Read the model definition and answer for the solid it produces. Units are mm, in the model's axes. Face numbers are marked on the shaded views. A direction names the side the tool comes from. Coordinates: 2 decimals unless noted, no trailing zeros. Loops run counter-clockwise (first coordinate to the right, second up) from the corner with the lowest first, then second, coordinate; pieces in that order, holes last.
Autodesk Fusion 360 part; units mm, degrees
sketch "草图1" plane through (0, 0, 0) normal (0, 0, 1) x (1, 0, 0)
  line L0 (-83.7376, 48.3346) -> (-83.7376, -57.8018)
  line L1 (100, -57.8018) -> (-83.7376, -57.8018)
  line L2 (99.9425, 14.822) -> (-83.7376, 48.3346)
  line L3 (99.9425, 14.822) -> (99.9425, -57.8018)
  line L4 (-75.3044, 2.9706) -> (90.6956, 2.9706)
  line L5 (90.6956, 2.9706) -> (90.6956, -51.4889)
  line L6 (90.6956, -51.4889) -> (-75.3044, -51.4889)
  line L7 (-75.3044, -51.4889) -> (-75.3044, 2.9706)
  dimension "d1" = 166
extrude "拉伸1" add sketch "草图1" along normal blind 20 contours L0 L1 L2 L3 | L4 L5 L6 L7
sketch "草图2" plane through (0, 0, 20) normal (0, 0, 1) x (-1, 0, 0)
  line L0 (83.7376, -48.3346) -> (83.7376, 57.8018)
  line L1 (83.7376, 57.8018) -> (-99.9425, 57.8018)
  line L2 (-99.9425, 57.8018) -> (-99.9425, -14.822)
  line L3 (-99.9425, -14.822) -> (83.7376, -48.3346)
  line L4 (75, -5) -> (-90, -5)
  line L5 (-90, -5) -> (-90, 50)
  line L6 (-90, 50) -> (75, 50)
  line L7 (75, 50) -> (75, -5)
extrude "拉伸2" cut sketch "草图2" against normal blind 15 contours L4 L5 L6 L7
sketch "草图3" plane through (0, 0, 20) normal (0, 0, 1) x (-1, 0, 0)
  line L0 (-90, -5) -> (-90, 50)
  line L1 (-90, 50) -> (75, 50)
  line L2 (75, 50) -> (75, -5)
  line L3 (75, -5) -> (-90, -5)
  line L4 (83.7376, -48.3346) -> (83.7376, 57.8018)
  line L5 (83.7376, 57.8018) -> (-99.9425, 57.8018)
  line L6 (-99.9425, 57.8018) -> (-99.9425, -14.822)
  line L7 (-99.9425, -14.822) -> (83.7376, -48.3346)
  line L8 (67.985, -5) -> (60.985, -5)
  line L9 (60.985, -5) -> (60.985, 26)
  line L10 (60.985, 26) -> (67.985, 26)
  line L11 (67.985, 26) -> (67.985, -5)
  line L12 (67.985, -5) -> (60.985, -5)
  line L13 (67.985, 26) -> (67.985, -5)
  line L14 (60.985, 26) -> (67.985, 26)
  line L15 (60.985, -5) -> (60.985, 26)
  line L16 (55.5549, 26) -> (55.5549, -5)
  line L17 (55.5549, -5) -> (48.5549, -5)
  line L18 (48.5549, -5) -> (48.5549, 26)
  line L19 (48.5549, 26) -> (55.5549, 26)
  line L20 (55.5549, 26) -> (55.5549, -5)
  line L21 (48.5549, 26) -> (55.5549, 26)
  line L22 (48.5549, -5) -> (48.5549, 26)
  line L23 (55.5549, -5) -> (48.5549, -5)
  line L24 (36.7829, -5) -> (29.7829, -5)
  line L25 (36.7829, 26) -> (36.7829, -5)
  line L26 (29.7829, 26) -> (36.7829, 26)
  line L27 (29.7829, -5) -> (29.7829, 26)
  line L28 (24.3528, 26) -> (24.3528, -5)
  line L29 (17.3528, 26) -> (24.3528, 26)
  line L30 (17.3528, -5) -> (17.3528, 26)
  line L31 (24.3528, -5) -> (17.3528, -5)
  line L32 (11.4154, 26) -> (11.4154, -5)
  line L33 (4.4154, -5) -> (4.4154, 26)
  line L34 (11.4154, -5) -> (4.4154, -5)
  line L35 (4.4154, 26) -> (11.4154, 26)
  line L36 (-52.6472, -5) -> (-59.6472, -5)
  line L37 (-21.4451, 26) -> (-21.4451, -5)
  line L38 (-9.015, -5) -> (-16.015, -5)
  line L39 (-28.4451, 26) -> (-21.4451, 26)
  line L40 (-28.4451, 26) -> (-21.4451, 26)
  line L41 (-40.2171, 26) -> (-40.2171, -5)
  line L42 (-40.2171, -5) -> (-47.2171, -5)
  line L43 (-72.5846, -5) -> (-72.5846, 26)
  line L44 (-47.2171, 26) -> (-40.2171, 26)
  line L45 (-47.2171, -5) -> (-47.2171, 26)
  line L46 (-52.6472, 26) -> (-52.6472, -5)
  line L47 (-65.5846, 26) -> (-65.5846, -5)
  line L48 (-9.015, 26) -> (-9.015, -5)
  line L49 (-16.015, 26) -> (-9.015, 26)
  line L50 (-21.4451, -5) -> (-28.4451, -5)
  line L51 (-28.4451, -5) -> (-28.4451, 26)
  line L52 (-16.015, -5) -> (-16.015, 26)
  line L53 (-28.4451, -5) -> (-28.4451, 26)
  line L54 (-9.015, -5) -> (-16.015, -5)
  line L55 (-16.015, 26) -> (-9.015, 26)
  line L56 (-72.5846, 26) -> (-65.5846, 26)
  line L57 (-65.5846, -5) -> (-72.5846, -5)
  line L58 (-21.4451, 26) -> (-21.4451, -5)
  line L59 (-9.015, 26) -> (-9.015, -5)
  line L60 (-21.4451, -5) -> (-28.4451, -5)
  line L61 (-59.6472, 26) -> (-52.6472, 26)
  line L62 (-59.6472, -5) -> (-59.6472, 26)
  line L63 (-16.015, -5) -> (-16.015, 26)
  line L64 (-82.7432, 26.3749) -> (-82.7432, -4.6251)
  line L65 (-89.7432, 26.3749) -> (-82.7432, 26.3749)
  line L66 (-89.7432, -4.6251) -> (-89.7432, 26.3749)
  line L67 (-82.9307, -4.8125) -> (-89.9307, -4.8125)
  point P0 (-77, 0)
  dimension "d6" = 7
  dimension "d7" = 31
  dimension "d8" = 7
  dimension "d9" = 31
  dimension "d10" = 7
  dimension "d11" = 31
  dimension "d12" = 7
  dimension "d13" = 31
  dimension "d14" = 7
  dimension "d15" = 31
  dimension "d16" = 31
  dimension "d17" = 7
  dimension "d18" = 31
  dimension "d19" = 7
  dimension "d22" = -77
  dimension "d23" = 0
  dimension "d24" = 7
  dimension "d25" = 31
  dimension "d26" = 7
extrude "拉伸3" add sketch "草图3" against normal blind 15 contours L3 L43 L47 L56 L57 | L3 L36 L46 L61 L62 | L3 L8 L9 L10 L11 L12 L13 L14 L15 | L3 L41 L42 L44 L45 | L3 L16 L17 L18 L19 L20 L21 L22 L23 | L3 L37 L39 L40 L50 L51 L53 L58 L60 | L3 L24 L25 L26 L27 | L3 L38 L48 L49 L52 L54 L55 L59 L63 | L3 L28 L29 L30 L31 | L3 L32 L33 L34 L35
sketch "草图4" plane through (0, 0, 20) normal (0, 0, 1) x (-1, 0, 0)
  line L0 (-90, -5) -> (-90, 50)
  line L1 (-90, 50) -> (75, 50)
  line L2 (75, 50) -> (75, -5)
  line L3 (75, -5) -> (67.985, -5)
  line L4 (67.985, -5) -> (67.985, 26)
  line L5 (67.985, 26) -> (60.985, 26)
  line L6 (60.985, 26) -> (60.985, -5)
  line L7 (60.985, -5) -> (55.5549, -5)
  line L8 (55.5549, -5) -> (55.5549, 26)
  line L9 (55.5549, 26) -> (48.5549, 26)
  line L10 (48.5549, 26) -> (48.5549, -5)
  line L11 (48.5549, -5) -> (36.7829, -5)
  line L12 (36.7829, -5) -> (36.7829, 26)
  line L13 (36.7829, 26) -> (29.7829, 26)
  line L14 (29.7829, 26) -> (29.7829, -5)
  line L15 (29.7829, -5) -> (24.3528, -5)
  line L16 (24.3528, -5) -> (24.3528, 26)
  line L17 (24.3528, 26) -> (17.3528, 26)
  line L18 (17.3528, 26) -> (17.3528, -5)
  line L19 (17.3528, -5) -> (11.4154, -5)
  line L20 (11.4154, -5) -> (11.4154, 26)
  line L21 (11.4154, 26) -> (4.4154, 26)
  line L22 (4.4154, 26) -> (4.4154, -5)
  line L23 (4.4154, -5) -> (-9.015, -5)
  line L24 (-9.015, -5) -> (-9.015, 26)
  line L25 (-9.015, 26) -> (-16.015, 26)
  line L26 (-16.015, 26) -> (-16.015, -5)
  line L27 (-16.015, -5) -> (-21.4451, -5)
  line L28 (-21.4451, -5) -> (-21.4451, 26)
  line L29 (-21.4451, 26) -> (-28.4451, 26)
  line L30 (-28.4451, 26) -> (-28.4451, -5)
  line L31 (-28.4451, -5) -> (-40.2171, -5)
  line L32 (-40.2171, -5) -> (-40.2171, 26)
  line L33 (-40.2171, 26) -> (-47.2171, 26)
  line L34 (-47.2171, 26) -> (-47.2171, -5)
  line L35 (-47.2171, -5) -> (-52.6472, -5)
  line L36 (-52.6472, -5) -> (-52.6472, 26)
  line L37 (-52.6472, 26) -> (-59.6472, 26)
  line L38 (-59.6472, 26) -> (-59.6472, -5)
  line L39 (-59.6472, -5) -> (-65.5846, -5)
  line L40 (-65.5846, -5) -> (-65.5846, 26)
  line L41 (-65.5846, 26) -> (-72.5846, 26)
  line L42 (-72.5846, 26) -> (-72.5846, -5)
  line L43 (-72.5846, -5) -> (-90, -5)
  line L44 (83.7376, -48.3346) -> (83.7376, 57.8018)
  line L45 (83.7376, 57.8018) -> (-99.9425, 57.8018)
  line L46 (-99.9425, 57.8018) -> (-99.9425, -14.822)
  line L47 (-99.9425, -14.822) -> (83.7376, -48.3346)
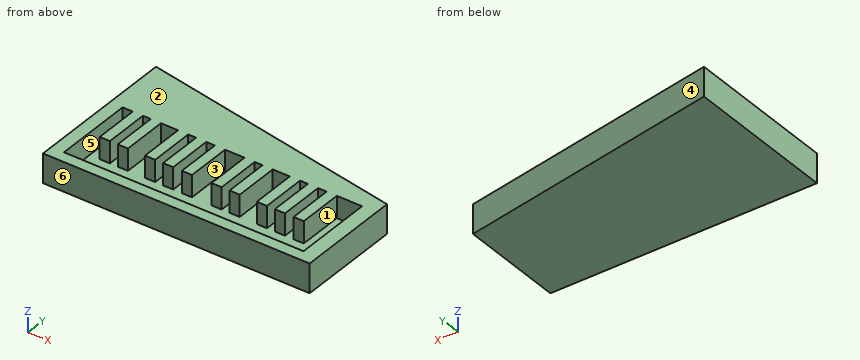
Q1. A cutting plane is placed at C-C (y = 25). Give the vertices of the cut face in (x, z), then the cut area to 3 significant figures.
Findings below:
outline: (-83.74, 0) - (44.16, 0) - (44.16, 20) - (-83.74, 20) - close
area: 2,560 mm2
Q2. A flat-ended cylindrical pin translates along its axis: pin 1 Ø1.5 at (x, z) = (-27.5, 5) entering from +Y. Find the tip coordinate at first contact, or state that the pin passes through.
Findings below:
pin 1: stops at y = 38.21
Q3. Which of the six approach directions +Z, -Z, +X, -X, +Y, -Y give full straight-line access (tool end or side, diameter ignored) to the marked faces 1 and 2?
Findings below:
face 1: +Z
face 2: +Z, +X, -X, +Y, -Y
Q4. Straight lines are drawn through the part: probe 1 along X at (y, z) = (-48, 5.25); probe 2 along Z at (x, y) = (38, 2.5); probe 3 along Y at (x, z) = (65.5, 18.75). For each, find the intervals that lie inside material, in ascending order.
Findings below:
probe 1: x = -83.74 to -75, 90 to 99.94
probe 2: z = 0 to 5
probe 3: y = -57.8 to -50, 5 to 21.11
Q5. A cutting plane is placed at B-B (x = -32). Give the vertices of the cut face in (y, z).
Findings below:
outline: (-57.8, 0) - (38.9, 0) - (38.9, 20) - (-26, 20) - (-26, 5) - (-50, 5) - (-50, 20) - (-57.8, 20) - close
Q6. Determine the mould class of the marked faces 3, 4, 5 and 6 for opening direction X: +X half, -X half, draft (parallel to the pull), parting line (faces both ways), or undercut.
Findings below:
face 3: undercut
face 4: +X half
face 5: undercut
face 6: draft
Q7. A cutting plane is placed at A-A (y = -42). Give the vertices of the cut face in (x, z).
Findings below:
outline: (-83.74, 0) - (99.94, 0) - (99.94, 20) - (90, 20) - (90, 5) - (-75, 5) - (-75, 20) - (-83.74, 20) - close
